```python
from build123d import *

# Parameters (mm, degrees)
SKETCH1_R           = 4
BOSS_EXTRUDE1_DEPTH = 20
SKETCH2_R           = 2.75
CUT_EXTRUDE1_DEPTH  = 10


with BuildPart() as part:
    # Sketch1 → Boss-Extrude1 (new body)
    with BuildSketch(Plane(origin=(0, 0, 0), x_dir=(1, 0, 0), z_dir=(0, 1, 0))):
        Polygon((0, 0), (0, 36), (6, 36), (6, 26), (22, 26), (22, 10), (6, 10), (6, 0), align=None)
        with Locations(Location((14, 18, 0), (0, 0, 270))):
            Circle(SKETCH1_R, mode=Mode.SUBTRACT)
    extrude(amount=BOSS_EXTRUDE1_DEPTH)

    # Sketch2 → Cut-Extrude1 (cut)
    with BuildSketch(Plane(origin=(6, 0, 0), x_dir=(0, 0, -1), z_dir=(1, 0, 0))):
        with Locations((5, 10)):
            Circle(SKETCH2_R)
        with Locations((31, 10)):
            Circle(SKETCH2_R)
    extrude(amount=-CUT_EXTRUDE1_DEPTH, mode=Mode.SUBTRACT)


solid = part.part
```
The listing builds one solid part. Answer for the finished solid, in the listing's coordinates (mm). A direction names the side the tool comes from. Give positions to 0.01 mm unless a question says otherwise; leave off trailing zeros. Loops run counter-clockwise (first coordinate to the right, second up) from the corner with the lowest first, then second, coordinate; pieces in that order, holes last. Notation, with made-up numbers: (-8, -9) - (19, -9) arc R22 ccw to (19, 6) - close; hole circle Ø11 at (56.5, -17). An arc over 180 degrees is marked (long way). Answer as CSV lines item,"result". Start each with the question number.
Item 1: A cutting plane is placed at B-B on z = -18. Determine the outline of the cut face in (x, y).
Item 2: The mould has two halves that part along Z. Classify faces 3 (the face through (14, 10, -26)), 4 (the face through (14, 10, -10)), 5 (the face through (3.042, 10.121, -28.253)), 6 (the face through (6, 7.6, -2.8)): +Z half, -Z half, draft (parallel to the pull), parting line (faces both ways), or undercut.
Item 3: Find the intervals of material crossed by line 1 (Y direction, x = 4.7, z = -5); line 2 (X direction, y = 9.25, z = -18); line 3 (Z direction, x = 9, y = 10), in increasing order. Write a range as from..to.
Item 4: For faces 1 (the face through (6, 7.6, -28.8)), 2 (the face through (0, 10, -18)), determine the directions among +Z, -Z, +X, -X, +Y, -Y from which every point of the face is accessible in a straight line to the end or side of a thin tool.
Item 5: A cutting plane is placed at D-D on y = 15. Determine the outline of the cut face in (x, z).
Item 6: Each of these flat-tipped pins is pushed along its axis until it touches: pin 1 (3 mm diameter, centred on x = 10, y = 12.5, fed in from -Z); pin 2 (8 mm diameter, centred on x = 11.5, y = 8, fed in from +Z); pin 3 (7 mm diameter, centred on y = 10, z = -5, fed in from +X). Where does it stop, or does it pass through?
Item 7: A cutting plane is placed at A-A on y = 10. Determine the outline of the cut face in (x, z), then the cut area to 3 significant figures.
Item 8: A cutting plane is placed at C-C on x = 14. Determine the outline of the cut face in (y, z), then the cut area to 3 significant figures.
Found:
1,outline,"(0, 0) - (10, 0) - (10, 20) - (0, 20) - close; (18, 0) - (22, 0) - (22, 20) - (18, 20) - close"
2,face 3,"-Z half"
2,face 4,"+Z half"
2,face 5,"undercut"
2,face 6,"draft"
3,line 1,"y = 0..7.25, 12.75..20"
3,line 2,"x = 0..10, 18..22"
3,line 3,"z = -26..-10"
4,face 1,"-Z, +X, +Y, -Y"
4,face 2,"+Z, -Z, -X, +Y, -Y"
5,outline,"(0, -36) - (6, -36) - (6, -26) - (22, -26) - (22, -10) - (6, -10) - (6, 0) - (0, 0) - close; hole circle Ø8 at (14, -18)"
6,pin 1,"stops at z = -26"
6,pin 2,"stops at z = -10"
6,pin 3,"stops at x = 6"
7,outline,"(0, -36) - (6, -36) - (6, -33.75) - (0, -33.75) - close; (0, -28.25) - (6, -28.25) - (6, -26) - (22, -26) - (22, -10) - (6, -10) - (6, -7.75) - (0, -7.75) - close; (0, -2.25) - (6, -2.25) - (6, 0) - (0, 0) - close; hole circle Ø8 at (14, -18)"
7,area,"356 mm^2"
8,outline,"(0, -26) - (20, -26) - (20, -22) - (0, -22) - close; (0, -14) - (20, -14) - (20, -10) - (0, -10) - close"
8,area,"160 mm^2"
